Build history of the part. All positions in model axes, mm. Face numbers are marked on the shaded views. A direction names the side the tool comes from. Give positions to 0.01 mm unless a question says otherwise; leave off trailing zeros. Loops run counter-clockwise (first coordinate to the right, second up) from the corner with the lowest first, then second, coordinate; pieces in that order, holes last. Notation, with made-up numbers: M -16,32.5 L 0,32.5 A25 ccw 0,52.5 Z; hole C 64,60 d1. An arc over 180 degrees is marked long. Answer as a JSON object with one key per item and string values. Group by question number.
1. Drop flat-ended pins along their axis: pin 1 Ø12 at (x, z) = (87.5, 33.5) entering from -Y; pin 2 Ø4 at (y, z) = (-47.5, 7) entering from -X; pin 3 Ø6 at (x, z) = (62, 39) entering from -Y. Give the stop position or say it passes through.
2. Mould opens along X. For the marked faces 3, 4 and 5 say: released by +X, released by -X, zero draft, split by the parting line, or undercut.
3. Slice it at C-C (z = 16). List the corners of the cut face in (x, y).
4. 3-axis set-ups, long thin cutter, end or side, ignore diameter. For the marked faces 1 and 2: which of +Z, -Z, +X, -X, +Y, -Y reach the whole face in a straight line?
5. Drill centre lines: line 1 along Y through (x, z) = (0, 1.15) (3 decimals); line 2 along Y through (x, z) = (0, 35.5); line 3 along Z through (x, y) = (60, -97). Where is each one in solid material? Low to high. Write a range as [from, to].
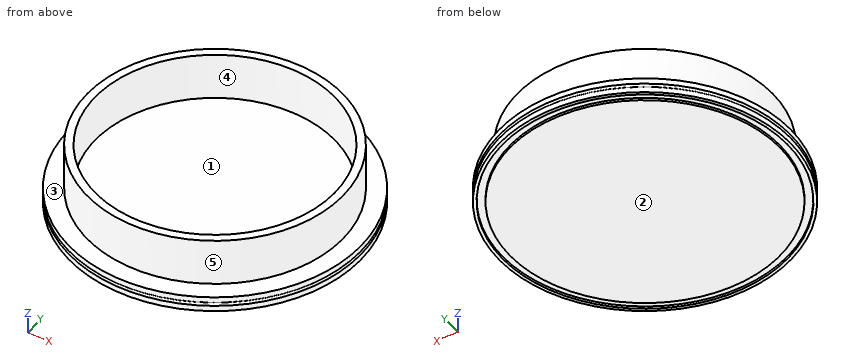
from build123d import *


with BuildPart() as part:
    # Sketch1 → Base-Revolve (revolve)
    with BuildSketch(Plane(origin=(0, 0, 0), x_dir=(0, 0, -1), z_dir=(1, 0, 0)), mode=Mode.PRIVATE) as base_revolve_sk:
        with BuildLine():
            Line((-4.585786438, 115.874999992), (0, 115.874999992))
            Line((0, 115.874999992), (0, 113.374999974))
            Line((0, 113.374999974), (-2, 113.374999974))
            Line((-2, 113.374999974), (-2, 107.374999974))
            Line((-2, 107.374999974), (0, 107.374999974))
            Line((0, 107.374999974), (0, 0))
            Line((0, 0), (-12, 0))
            Line((-12, 0), (-12, 95.25))
            Line((-12, 95.25), (-49.538490201, 95.25))
            Line((-49.538490201, 95.25), (-49.538490201, 101.6))
            Line((-49.538490201, 101.6), (-12, 101.6))
            Line((-12, 101.6), (-12, 115.874999992))
            Line((-12, 115.874999992), (-7.414213562, 115.874999992))
            ThreePointArc((-7.414213562, 115.874999992), (-6, 114.874999992), (-4.585786438, 115.874999992))
        make_face()
    revolve(base_revolve_sk.sketch.rotate(Axis((0, 0, 12), (0, 0, -1)), 90), axis=Axis((0, 0, 12), (0, 0, -1)))


solid = part.part
Established:
{
 "1": {"pin 1": "stops at y = -60.67", "pin 2": "stops at x = -106.55", "pin 3": "stops at y = -82.71"},
 "2": {"face 3": "zero draft", "face 4": "undercut", "face 5": "split by the parting line"},
 "3": {"outline": "C 0,0 d203.2; hole C 0,0 d190.5"},
 "4": {"face 1": "+Z", "face 2": "-Z, +X, -X, +Y, -Y"},
 "5": {"line 1": "y = [-115.875, -113.375], [-107.375, 107.375], [113.375, 115.875]", "line 2": "y = [-101.6, -95.25], [95.25, 101.6]", "line 3": "z = [0, 12]"}
}
